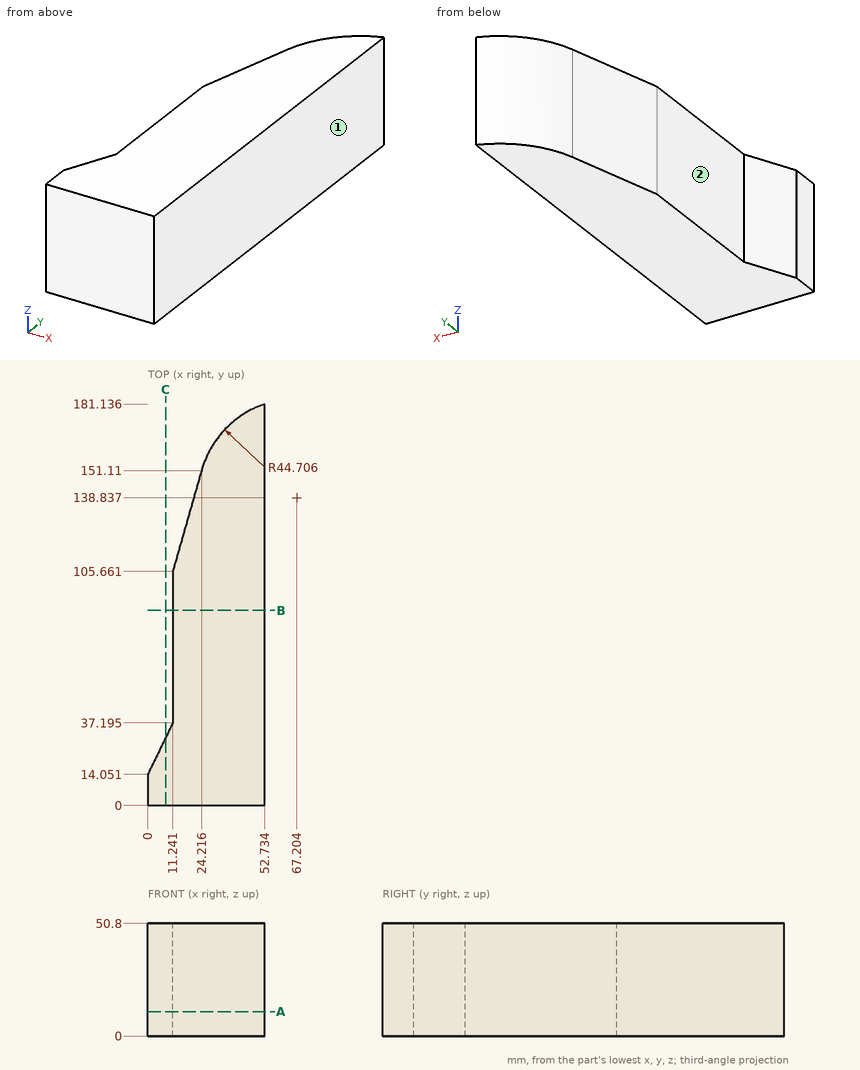
Can you work these out from the drawing? Everything is in mm from the part's minimum corner. A direction names the side the tool comes from. Give positions to 0.01 mm unless a question says otherwise; leave off trailing zeros. Write each loop counter-clockwise with the first axis right and the second up, starting at its lowest first coordinate (ties: lowest second). Pieces come first, ordered by that corner, then holes. Notation, with made-up numbers: M 81.25,19 L 140.25,19 A15 ccw 140.25,34 Z; hole C 64.5,86.25 d1. An arc over 180 degrees is marked long. Answer in a Markdown table with one row per item. Add a question column.
Item 1: Please list where these lines run through material, in increasing order: L1, parallel to X at y = 72, z = 36; L2, parallel to X at y = 172, z = 38 (1 decimal); L3, parallel to Y at x = 39, z = 23.5.
Item 2: Imagine slicing it at C-C, the plane x = 8. Write out the boundary of the cut face in (y, z), plus the area to 3 significant figures.
Item 3: On a 3-axis mill with a long thin cutter (end or side, diameter ignored), from which of +Z, -Z, +X, -X, +Y, -Y can I reach the whole of each face in a straight line? I mean the marked faces 1 and 2. Say none if no direction works.
Item 4: Imagine slicing it at B-B, the plane y = 88. Write out the boundary of the cut face in (x, z), plus the area to 3 significant figures.
Item 5: For pin 1 Ø6 at (y, z) = (153, 19) entering from -X; pin 2 Ø8 at (x, z) = (42, 26.5) entering from +Y (1 decimal); pin 3 Ø4 at (y, z) = (86, 32.5) entering from -X, each with a flat end and sliding along its axis, tell me the tip position at first contact or that it passes through.
Item 6: Imagine slicing it at A-A, the plane z = 11. Write out the boundary of the cut face in (x, y) (1 decimal).
Evaluation:
| question | item | result |
|---|---|---|
| 1 | L1 | x = 11.24 to 52.73 |
| 1 | L2 | x = 37.2 to 52.7 |
| 1 | L3 | y = 0 to 173.52 |
| 2 | outline | M 0,0 L 30.52,0 L 30.52,50.8 L 0,50.8 Z |
| 2 | area | 1,550 mm² |
| 3 | face 1 | +Z, -Z, +X, +Y, -Y |
| 3 | face 2 | +Z, -Z, -X, +Y |
| 4 | outline | M 11.24,0 L 52.73,0 L 52.73,50.8 L 11.24,50.8 Z |
| 4 | area | 2,110 mm² |
| 5 | pin 1 | stops at x = 23.9 |
| 5 | pin 2 | stops at y = 178.2 |
| 5 | pin 3 | stops at x = 11.24 |
| 6 | outline | M 0,0 L 52.7,0 L 52.7,181.1 A44.7 ccw 24.2,151.1 L 11.2,105.7 L 11.2,37.2 L 0,14.1 Z |
